Answer from the drawing. Dimensions are ordinates in mm from the lowest x, y and z of the part. Coordinates: 2 decimals unless noted, no trailing zeros. Order: outer loops, then holes, each group sorted by start corner. A loop starts at its lowest first (then second) coordinate and runs counter-clockwise, first axis right, second up. Notation, with made-up numbers: (37, 57.25) - (92, 57.25) arc R12 ccw to (92, 64.25) - close; hole circle Ø4 at (3.5, 0.25). An arc over 180 degrees is marked (long way). Answer as a JSON object with one key per item and string values. Group by question number.
1) Find the intervals of material crossed by line 1 along Y through (x, z) = (20, 22); line 2 along X through (y, z) = (3.5, 27.5); line 3 along Z through (x, y) = (8.5, 3.7) (1 decimal), in increasing order.
2) Section B-B (y = 2.85) is taken. Give the vertices of the cut face in (x, z), plus the area to 4 significant figures.
3) Section D-D (z = 26.5) is taken. Give the vertices of the cut face in (x, y).
4) Section A-A (x = 12.5) is taken. Give the vertices of the cut face in (y, z).
5) Each of these flat-tipped pins is pushed along its axis until it touches: P1, Ø1.7, axis at y = 3, z = 30.5, coming from the -X side; P2, Ø1.7, axis at y = 3, z = 28.5, coming from the +X side; P3, Ø1, axis at x = 22, z = 27.5, coming from the +Y side. Where does it stop, or does it pass through?
6) Section C-C (z = 35.5) is taken. Give the vertices of the cut face in (x, y).
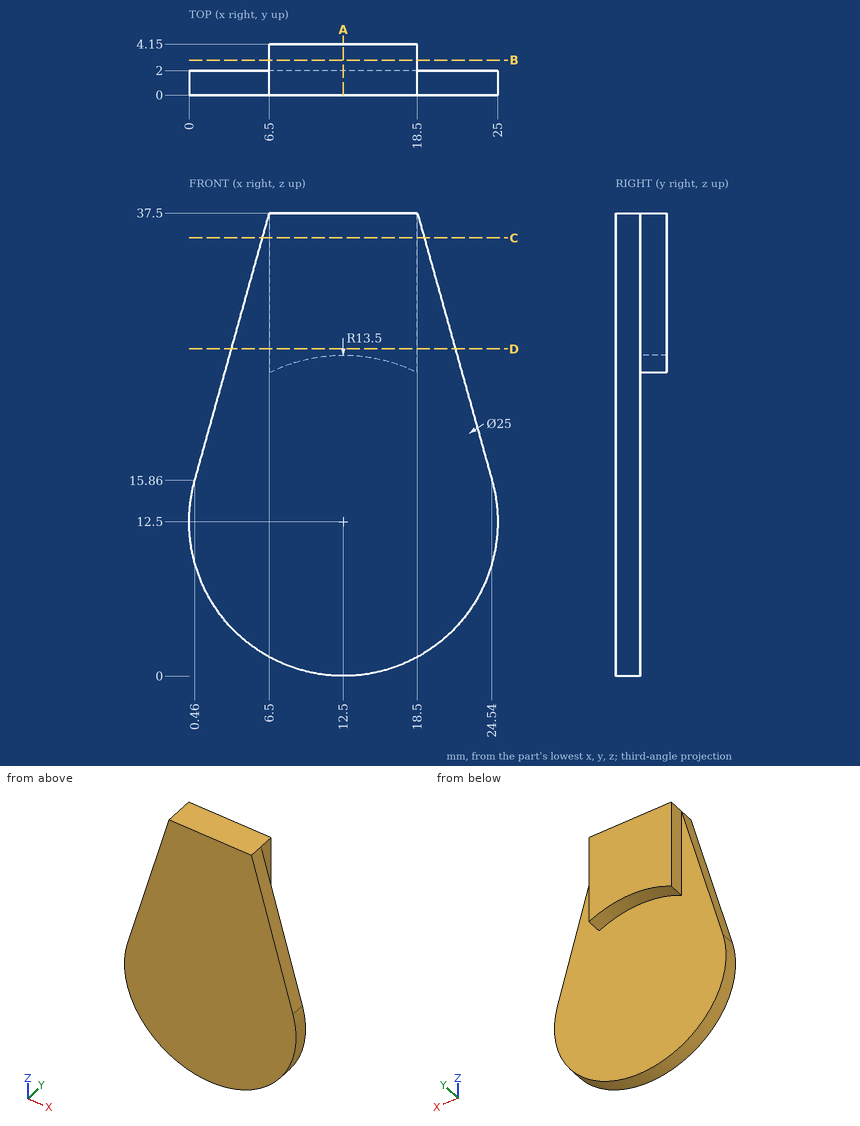
Report:
{
 "1": {"line 1": "y = 0 to 2", "line 2": "x = 6.5 to 18.5", "line 3": "z = 25.4 to 37.5"},
 "2": {"outline": "(6.5, 24.59) arc R13.5 cw to (18.5, 24.59) - (18.5, 37.5) - (6.5, 37.5) - close", "area": "143.5 mm²"},
 "3": {"outline": "(3.43, 0) - (21.57, 0) - (21.57, 2) - (18.5, 2) - (18.5, 4.15) - (6.5, 4.15) - (6.5, 2) - (3.43, 2) - close"},
 "4": {"outline": "(0, 0) - (2, 0) - (2, 26) - (4.15, 26) - (4.15, 37.5) - (0, 37.5) - close"},
 "5": {"P1": "stops at x = 6.5", "P2": "stops at x = 18.5", "P3": "passes through"},
 "6": {"outline": "(5.94, 0) - (19.06, 0) - (19.06, 2) - (18.5, 2) - (18.5, 4.15) - (6.5, 4.15) - (6.5, 2) - (5.94, 2) - close"}
}
